Here's how the part is built. I have some questions about the finished solid (model axes, mm). A direction names the side the tool comes from. Give positions to 0.01 mm unless a question says otherwise; leave off trailing zeros. Loops run counter-clockwise (first coordinate to the right, second up) from the corner with the lowest first, then second, coordinate; pieces in that order, holes last.
Q1. If we section it at B-B (y = 5.75): Please give me the cut outline in (x, z).
Q2. For faces 5 (the face through (-1, 3, 0)), 6 (the face through (22, 1, 17.5)), 7 (the face through (17, 6, 5)), which set-ups out of +Z, -Z, +X, -X, +Y, -Y let a thin tool reach every point of the face, with its end or its side?
Q3. If we section it at A-A (y = 1): Please give me the cut outline in (x, z), plus the area to 3 significant figures.
Q4. If we section it at D-D (y = 10): Please give me the cut outline in (x, z), plus the area to 3 significant figures.
Q5. If we section it at C-C (z = 0): Please give me the cut outline in (x, y), plus the area to 3 significant figures.
Q6. We'd pull the mould along X, two halves only. Please class faces 1 (the face through (17, 6, 17.5)), 2 (the face through (15.13, 8.07, 18.77)), 3 (the face through (-24, 3, 4)), 4 (the face through (-25.237, 1.479, -0.198)): +X half, -X half, draft (parallel to the pull), parting line (faces both ways), or undercut.
Q7. Will these pins go through, and if not, where does the flat tip stop? P1, Ø1.5, axis at y = 1.5, z = -14, coming from the +X side; P2, Ø6, axis at y = 1.5, z = -5.5, coming from the -X side; P3, Ø5, axis at x = -18.5, z = -3.5, coming from the +Y side.
Q8. I need wall thicknesses on line 1 (Z direction, x = 17.5, y = 4); line 2 (X direction, y = 2.3, z = 0); line 3 (X direction, y = 5.25, z = 0). Which ranges of each line are inside material? Lowest first, please.
from build123d import *

# Parameters (mm, degrees)
BOSS_EXTRUDE1_DEPTH = 3
BOSS_EXTRUDE3_DEPTH = 2.5
LPATTERN2_COUNT     = 4
LPATTERN2_PITCH     = 12.5
SKETCH3_R           = 11.65
SKETCH3_R_2         = 8.15
BOSS_EXTRUDE4_DEPTH = 6
SKETCH4_R           = 4.5
CUT_EXTRUDE2_DEPTH  = 14
FILLET1_R           = 2
FILLET2_R           = 2


with BuildPart() as part:
    # Sketch1 → Boss-Extrude1 (new body)
    with BuildSketch(Plane(origin=(0, 0, 0), x_dir=(1, 0, 0), z_dir=(0, 1, 0))):
        with BuildLine():
            Line((20, 17.5), (23.592842073, 17.5))
            Line((23.592842073, 17.5), (23.592842073, 12.5))
            Line((23.592842073, 12.5), (19.944472227, 12.5))
            Line((19.944472227, 12.5), (20.019420438, 7.500018858))
            Line((20.019420438, 7.500018858), (23.612262511, 7.500018858))
            Line((23.612262511, 7.500018858), (23.612262511, 2.500018858))
            Line((23.612262511, 2.500018858), (20.019420438, 2.500018858))
            Line((20.019420438, 2.500018858), (20.038840876, -2.499962285))
            Line((20.038840876, -2.499962285), (23.63168295, -2.499962285))
            Line((23.63168295, -2.499962285), (23.63168295, -7.499962285))
            Line((23.63168295, -7.499962285), (20.038840876, -7.499962285))
            Line((20.038840876, -7.499962285), (20.058261315, -12.499943427))
            Line((20.058261315, -12.499943427), (23.651103388, -12.499943427))
            Line((23.651103388, -12.499943427), (23.651103388, -17.499943427))
            Line((23.651103388, -17.499943427), (20.058261315, -17.499943427))
            Line((20.058261315, -17.499943427), (20, -20))
            Line((20, -20), (-20, -20))
            ThreePointArc((-20, -20), (-40, 0), (-20, 20))
            Line((-20, 20), (20, 20))
            Line((20, 20), (20, 17.5))
        make_face()
    extrude(amount=BOSS_EXTRUDE1_DEPTH)

    # Sketch2 → Boss-Extrude3 (add)
    with BuildSketch(Plane.XY.offset(20)):
        Polygon((20.058261315, 3), (20.058261315, 13), (10.058261315, 3), align=None)
    boss_extrude3 = extrude(amount=-BOSS_EXTRUDE3_DEPTH)

    # LPattern2: Boss-Extrude3 ×4
    with Locations(*[Vector(-0.003884073, 0, -0.999992457) * (i * LPATTERN2_PITCH) for i in range(1, LPATTERN2_COUNT)]):
        add(boss_extrude3)

    # Sketch3 → Boss-Extrude4 (add)
    with BuildSketch(Plane(origin=(0, 3, 0), x_dir=(1, 0, 0), z_dir=(0, 1, 0))):
        with Locations((-20.741708838, 0)):
            Circle(SKETCH3_R)
        with Locations((-20.741708838, 0)):
            Circle(SKETCH3_R_2, mode=Mode.SUBTRACT)
    extrude(amount=BOSS_EXTRUDE4_DEPTH)

    # Sketch4 → Cut-Extrude2 (cut, through all)
    with BuildSketch(Plane(origin=(0, 0, 0), x_dir=(1, 0, 0), z_dir=(0, 1, 0))):
        with Locations((-20.741708838, 0)):
            Circle(SKETCH4_R)
    extrude(amount=CUT_EXTRUDE2_DEPTH, mode=Mode.SUBTRACT)

    # Fillet1
    fillet1_edges = [part.edges().sort_by_distance(p)[0] for p in [
        (-32.391708838, 3, 0),
    ]]
    fillet(fillet1_edges, radius=FILLET1_R)

    # Fillet2
    fillet2_edges = [part.edges().sort_by_distance(p)[0] for p in [
        (-32.391708838, 9, 0),
    ]]
    fillet(fillet2_edges, radius=FILLET2_R)


solid = part.part
Check sheet entries:
1. outline: circle Ø23.3 at (-20.74, 0); (12.66, -20) - (19.91, -20) - (19.91, -17.5) - (12.66, -17.5) - close; (12.71, -7.5) - (19.96, -7.5) - (19.96, -5) - (12.71, -5) - close; (12.76, 5) - (20.01, 5) - (20.01, 7.5) - (12.76, 7.5) - close; (12.81, 17.5) - (20.06, 17.5) - (20.06, 20) - (12.81, 20) - close; hole circle Ø16.3 at (-20.74, 0)
2. face 5: +Y
2. face 6: +Z, +X, +Y, -Y
2. face 7: +X, +Y
3. outline: (-20, -20) - (20, -20) - (20, -17.5) - (23.59, -17.5) - (23.59, -12.5) - (19.94, -12.5) - (20.02, -7.5) - (23.61, -7.5) - (23.61, -2.5) - (20.02, -2.5) - (20.04, 2.5) - (23.63, 2.5) - (23.63, 7.5) - (20.04, 7.5) - (20.06, 12.5) - (23.65, 12.5) - (23.65, 17.5) - (20.06, 17.5) - (20, 20) - (-20, 20) arc R20 ccw to start; hole circle Ø9 at (-20.74, 0)
3. area: 2,240 mm2
4. outline: (16.91, -20) - (19.91, -20) - (19.91, -17.5) - (16.91, -17.5) - close; (16.96, -7.5) - (19.96, -7.5) - (19.96, -5) - (16.96, -5) - close; (17.01, 5) - (20.01, 5) - (20.01, 7.5) - (17.01, 7.5) - close; (17.06, 17.5) - (20.06, 17.5) - (20.06, 20) - (17.06, 20) - close
4. area: 30.0 mm2
5. outline: (-40, 0) - (-25.24, 0) - (-25.24, 3) - (-28.89, 3) - (-28.89, 9) - (-30.39, 9) arc R2 ccw to (-32.39, 7) - (-32.39, 5) arc R2 cw to (-34.39, 3) - (-40, 3) - close; (-16.24, 0) - (20.03, 0) - (20.03, 3) - (-7.09, 3) arc R2 cw to (-9.09, 5) - (-9.09, 7) arc R2 ccw to (-11.09, 9) - (-12.59, 9) - (-12.59, 3) - (-16.24, 3) - close
5. area: 195 mm2
6. face 1: draft
6. face 2: -X half
6. face 3: undercut
6. face 4: undercut
7. P1: stops at x = 23.59
7. P2: stops at x = -39.84
7. P3: stops at y = 3
8. line 1: z = -20 to -17.5, -7.5 to -5, 5 to 7.5, 17.5 to 20
8. line 2: x = -40 to -25.24, -16.24 to 20.03
8. line 3: x = -32.39 to -28.89, -12.59 to -9.09
